```python
from build123d import *

# Parameters (mm, degrees)
SKETCH1_W           = 87.4
SKETCH1_H           = 39
BOSS_EXTRUDE1_DEPTH = 30
CUT_EXTRUDE1_START  = -4
CUT_EXTRUDE1_DEPTH  = 22
SKETCH3_W           = 30
SKETCH3_H           = 22
CUT_EXTRUDE2_DEPTH  = 66.80797824
SKETCH4_R           = 1.9
CUT_EXTRUDE3_DEPTH  = 15
SKETCH5_R           = 4
BOSS_EXTRUDE2_DEPTH = 6
SKETCH6_R           = 2.5
CUT_EXTRUDE4_DEPTH  = 10


with BuildPart() as part:
    # Sketch1 → Boss-Extrude1 (new body)
    with BuildSketch(Plane.XY):
        with Locations((0, 19.5)):
            Rectangle(SKETCH1_W, SKETCH1_H)
    extrude(amount=BOSS_EXTRUDE1_DEPTH)

    # Sketch2 → Cut-Extrude1 (cut)
    with BuildSketch(Plane.XY.offset(30).offset(CUT_EXTRUDE1_START)):
        with BuildLine():
            Line((-38.667900264, 0), (38.667900264, 0))
            Line((38.667900264, 0), (37.107871406, 4.560366948))
            ThreePointArc((37.107871406, 4.560366948), (33.096716485, 9.948855693), (26.7, 12))
            Line((26.7, 12), (-26.7, 12))
            ThreePointArc((-26.7, 12), (-33.096716485, 9.948855693), (-37.107871406, 4.560366948))
            Line((-37.107871406, 4.560366948), (-38.667900264, 0))
        make_face()
    extrude(amount=-CUT_EXTRUDE1_DEPTH, mode=Mode.SUBTRACT)

    # Sketch3 → Cut-Extrude2 (cut, through all)
    with BuildSketch(Plane.XY.offset(30)):
        Polygon((-43.7, 0), (-30.358721505, 39), (-43.7, 39), align=None)
        with Locations((0, 28)):
            Rectangle(SKETCH3_W, SKETCH3_H)
        Polygon((30.358721505, 39), (43.7, 0), (43.7, 39), align=None)
    extrude(amount=-CUT_EXTRUDE2_DEPTH, mode=Mode.SUBTRACT)

    # Sketch4 → Cut-Extrude3 (cut)
    with BuildSketch(Plane(origin=(0, 39, 0), x_dir=(1, 0, 0), z_dir=(0, 1, 0))):
        with Locations(Location((-20, -15, 0), (0, 0, 180))):
            Circle(SKETCH4_R)
        with Locations(Location((20, -15, 0), (0, 0, 180))):
            Circle(SKETCH4_R)
    extrude(amount=-CUT_EXTRUDE3_DEPTH, mode=Mode.SUBTRACT)

    # Sketch5 → Boss-Extrude2 (add)
    with BuildSketch(Plane.XY.offset(30)):
        with Locations(Location((25, 6, 0), (0, 0, 180))):
            Circle(SKETCH5_R)
        with Locations(Location((-25, 6, 0), (0, 0, 180))):
            Circle(SKETCH5_R)
    extrude(amount=BOSS_EXTRUDE2_DEPTH)

    # Sketch6 → Cut-Extrude4 (cut)
    with BuildSketch(Plane.XY.offset(36)):
        with Locations((25, 6)):
            Circle(SKETCH6_R)
        with Locations((-25, 6)):
            Circle(SKETCH6_R)
    extrude(amount=-CUT_EXTRUDE4_DEPTH, mode=Mode.SUBTRACT)


solid = part.part
```
Work out the finished part from the listing and answer in its coordinate system (mm). A direction names the side the tool comes from. Round coordinates to 2 decimals unless told otherwise and drop trailing zeros. Write each loop counter-clockwise with the first axis right and the second up, starting at its lowest first coordinate (ties: lowest second). Pieces come first, ordered by that corner, then holes. Notation, with made-up numbers: (-40, -33) -> (-28, -33) arc R13 cw to (-28, -19) -> close; hole circle Ø2 at (-22, 41.25). An arc over 180 degrees is marked (long way). Write each question's results on one line, items separated by ' | '.
Q1. Section A-A, the plane y = 28 is taken. Write down the section's boundary in (x, z), then the cut area to 3 significant figures.
Data:
outline: (-34.12, 0) -> (-15, 0) -> (-15, 30) -> (-34.12, 30) -> close; (15, 0) -> (34.12, 0) -> (34.12, 30) -> (15, 30) -> close; hole circle Ø3.8 at (-20, 15); hole circle Ø3.8 at (20, 15) | area: 1,120 mm^2
Q2. Determine the mould class of faces 1 (the flat face through (0, 17, 15)), 2 (the flat face through (-1, 15, 0)), 3 (the flat face through (20, 24, 15)), 4 (the flat face through (-1, 6, 4)) for opening direction Z: released by +Z, released by -Z, zero draft, split by the parting line, or undercut.
Data:
face 1: zero draft | face 2: released by -Z | face 3: undercut | face 4: undercut
Q3. Section D-D, the plane y = 7 is taken. Write down the section's boundary in (x, z).
Data:
outline: (-41.31, 0) -> (41.31, 0) -> (41.31, 30) -> (28.87, 30) -> (28.87, 36) -> (27.29, 36) -> (27.29, 26) -> (35.92, 26) -> (35.92, 4) -> (-35.92, 4) -> (-35.92, 26) -> (-27.29, 26) -> (-27.29, 36) -> (-28.87, 36) -> (-28.87, 30) -> (-41.31, 30) -> close; (-22.71, 26) -> (22.71, 26) -> (22.71, 36) -> (21.13, 36) -> (21.13, 30) -> (-21.13, 30) -> (-21.13, 36) -> (-22.71, 36) -> close
Q4. Straight lines are drawn through the part: line 1 along Z through (x, y) = (28.5, 2.5); line 2 along Y through (x, z) = (-25, 33); line 3 along X through (y, z) = (26, 16). For each, find the intervals that lie inside material, in ascending order. Write a range as [from, to].
Data:
line 1: [0, 4], [26, 30] | line 2: [2, 3.5], [8.5, 10] | line 3: [-34.81, -21.62], [-18.38, -15], [15, 18.38], [21.62, 34.81]
Q5. Flat-ended cylindrical pins translate along their axes: P1, Ø6.5, axis at x = 6.5, z = 9.5, coming from the -Y side; P2, Ø8, axis at y = 7, z = 7, coming from the +X side; P3, Ø11, axis at y = 26.5, z = 12.5, coming from the -X side. Find the tip coordinate at first contact, or state that the pin passes through.
Data:
P1: y = 12 | P2: x = 42.67 | P3: x = -36.52
Q6. Section B-B, the plane x = 25 is taken. Write down the section's boundary in (y, z).
Data:
outline: (0, 0) -> (39, 0) -> (39, 30) -> (10, 30) -> (10, 36) -> (8.5, 36) -> (8.5, 26) -> (12, 26) -> (12, 4) -> (0, 4) -> close; (0, 26) -> (3.5, 26) -> (3.5, 36) -> (2, 36) -> (2, 30) -> (0, 30) -> close
Q7. Which of the six approach directions +Z, -Z, +X, -X, +Y, -Y give full straight-line access (tool end or side, diameter ignored) to faces 5 (the flat face through (37.9, 2.25, 15.15)), 6 (the cylindrical face through (-26.84, 7.69, 31.07)), 7 (the flat face through (-15, 28, 15))?
Data:
face 5: -Y | face 6: +Z | face 7: +Z, -Z, +Y
Q8. Section C-C, the plane z = 25 is taken. Write down the section's boundary in (x, y), then the cut area to 3 significant figures.
Data:
outline: (-43.7, 0) -> (-38.67, 0) -> (-37.11, 4.56) arc R11 cw to (-26.7, 12) -> (26.7, 12) arc R11 cw to (37.11, 4.56) -> (38.67, 0) -> (43.7, 0) -> (30.36, 39) -> (15, 39) -> (15, 17) -> (-15, 17) -> (-15, 39) -> (-30.36, 39) -> close | area: 1,370 mm^2
